```python
from build123d import *

# Parameters (mm, degrees)
F0_R     = 4
F1_DEPTH = 4


with BuildPart() as f1:
    # F0 (on Front) → F1 (new body)
    with BuildSketch(Plane.XZ):
        Polygon((0, 220), (0, 0), (31.35714, 0), (31.35714, 12.080761), (113.539034, 89.704465), (100.003339, 107.905552), (31.35714, 56.855083), (31.35714, 220), align=None)
        with Locations((12.726834, 10)):
            Circle(F0_R, mode=Mode.SUBTRACT)
        with Locations((97.194239, 94.467405)):
            Circle(F0_R, mode=Mode.SUBTRACT)
        with Locations((12.726834, 210)):
            Circle(F0_R, mode=Mode.SUBTRACT)
    extrude(amount=F1_DEPTH)


solid = f1.part
```
Verification items for the finished model (mm, model axes). A direction names the side the tool comes from. Give positions to 0.01 mm unless a question says otherwise; leave off trailing zeros. Order: outer loops, then holes, each group sorted by start corner. A loop starts at its lowest first (then second) coordinate and runs counter-clockwise, first axis right, second up. Notation, with made-up numbers: (-18, 59.25) -> (5, 59.25) arc R7 ccw to (5, 67.25) -> close; hole circle Ø2 at (14.25, 77). An arc over 180 degrees is marked (long way). Use a Markdown table: item, result.
1) Section check A-A, the plane z = 210. Record the boundary of the cut face in (x, y), then the cut area to 3 significant figures.
Results:
| item | result |
|---|---|
| outline | (0, -4) -> (8.73, -4) -> (8.73, 0) -> (0, 0) -> close; (16.73, -4) -> (31.36, -4) -> (31.36, 0) -> (16.73, 0) -> close |
| area | 93.4 mm² |
2) Mould release check, pull along X, two halves, no side actions. Record for faces 1 (the cylindrical face through (12.206, -1.972, 213.966)), 2 (the cylindrical face through (8.73, -1.97, 10.18)), 3 (the flat face through (31, 0, 112)), 4 (the flat face through (31.357, -2, 6)): pulls with the +X half, pulls with the -X half, needs draft (parallel to the pull), parting line crosses it, or undercut.
Results:
| item | result |
|---|---|
| face 1 | undercut |
| face 2 | undercut |
| face 3 | needs draft |
| face 4 | pulls with the +X half |
3) Material ranges on probe 1 along X at (y, z) = (-1.85, 190.5); probe 2 along X at (y, z) = (-3.35, 91); probe 3 along Z at (x, y) = (14.5, -0.9), recorded low to high.
Results:
| item | result |
|---|---|
| probe 1 | 0 to 31.36 |
| probe 2 | 0 to 31.36, 77.27 to 95.2, 99.19 to 112.58 |
| probe 3 | 0 to 6.41, 13.59 to 206.41, 213.59 to 220 |
4) Tool access check on faces 5 (the flat face through (71.873, -1.972, 50.349)), 6 (the flat face through (66.161, -1.972, 82.738)). Record the directions out of +Z, -Z, +X, -X, +Y, -Y that give a thin tool (end or side, any length) a straight path to the whole face; none if there is none.
Results:
| item | result |
|---|---|
| face 5 | -Z, +X, +Y, -Y |
| face 6 | +Z, +Y, -Y |
5) Section check B-B, the plane x = 97. Record the boundary of the cut face in (y, z), then the cut area to 3 significant figures.
Results:
| item | result |
|---|---|
| outline | (-4, 74.08) -> (0, 74.08) -> (0, 90.47) -> (-4, 90.47) -> close; (-4, 98.46) -> (0, 98.46) -> (0, 105.67) -> (-4, 105.67) -> close |
| area | 94.4 mm² |
6) Depth check by flat-ended pin: pin 1 Ø1.5 at (x, y) = (55, -1) entering from +Z; pin 2 Ø12 at (x, z) = (49.5, 80.5) entering from -Y; pin 3 Ø9 at (x, z) = (12.73, 10) entering from +Y. Enter the tip coordinate at first touch or a pass-through.
Results:
| item | result |
|---|---|
| pin 1 | z = 75 |
| pin 2 | through |
| pin 3 | y = 0 |
7) Section check C-C, the plane y = -0.7. Record the boundary of the cut face in (x, z).
Results:
| item | result |
|---|---|
| outline | (0, 0) -> (31.36, 0) -> (31.36, 12.08) -> (113.54, 89.7) -> (100, 107.91) -> (31.36, 56.86) -> (31.36, 220) -> (0, 220) -> close; hole circle Ø8 at (12.73, 10); hole circle Ø8 at (12.73, 210); hole circle Ø8 at (97.19, 94.47) |
8) Section check D-D, the plane x = 77. Record the boundary of the cut face in (y, z), then the cut area to 3 significant figures.
Results:
| item | result |
|---|---|
| outline | (-4, 55.19) -> (0, 55.19) -> (0, 90.8) -> (-4, 90.8) -> close |
| area | 142 mm² |
